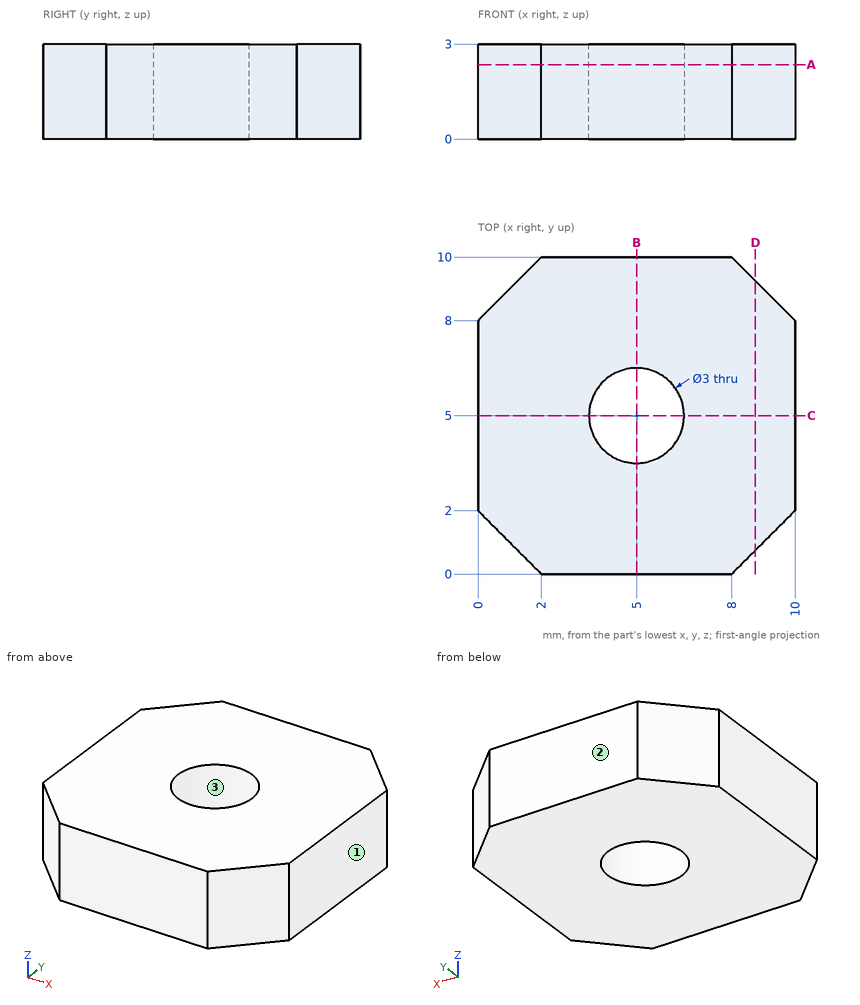
Input: dimensioned drawing with shaded views. Units: mm. Origin: part minimum x, y, z. Round coordinates to 2 decimals unless told otherwise and drop trailing zeros. Order: outer loops, then holes, each group sorted by start corner. A loop starts at its lowest first (then second) coordinate and runs counter-clockwise, first axis right, second up. Notation, with made-up numbers: M 33.25,10 L 71.25,10 A16 ccw 71.25,39 Z; hole C 66,56.5 d5. An arc over 180 degrees is marked long. Use one line per item in the form item = value. Start each with the question number.
Q1. Cut plane B-B (x = 5). Return loops of the section in (y, z), and give its area (3 significant figures).
Q2. Cut plane A-A (z = 2.35). Return loops of the section in (x, y), and give its area (3 significant figures).
Q3. Material intervals for line 1 (Y direction, x = 5, z = 1.3); line 2 (X direction, y = 3.75, z = 1.95); line 3 (X direction, y = 1, z = 0.75), sorted ascending. Write a range as [from, to].
Q4. Cut plane D-D (x = 8.75). Return loops of the section in (y, z).
Q5. Mould query, pull axis Y, two halves, no side actions, for the marked faces 1, 2 and 3. Classes: +Y half, -Y half, draft (parallel to the pull), parting line (faces both ways), or undercut.
Geometry results:
q1.outline = M 0,0 L 3.5,0 L 3.5,3 L 0,3 Z; M 6.5,0 L 10,0 L 10,3 L 6.5,3 Z
q1.area = 21.0 mm^2
q2.outline = M 0,2 L 2,0 L 8,0 L 10,2 L 10,8 L 8,10 L 2,10 L 0,8 Z; hole C 5,5 d3
q2.area = 84.9 mm^2
q3.line_1 = [0, 3.5], [6.5, 10]
q3.line_2 = [0, 4.17], [5.83, 10]
q3.line_3 = [1, 9]
q4.outline = M 0.75,0 L 9.25,0 L 9.25,3 L 0.75,3 Z
q5.face_1 = draft
q5.face_2 = +Y half
q5.face_3 = undercut
